Geometry check sheet. Reference: the model listing, model coordinates, mm. Face numbers are marked on the shaded views. A direction names the side the tool comes from. Coordinates: 2 decimals unless noted, no trailing zeros. Order: outer loops, then holes, each group sorted by start corner. A loop starts at its lowest first (then second) coordinate and runs counter-clockwise, first axis right, second up. Notation, with made-up numbers: (0.25, 82.25) -> (19.25, 82.25) arc R24 cw to (19.25, 108.25) -> close; hole circle Ø9 at (-32.5, 72). An arc over 180 degrees is marked (long way). Answer as CSV lines item,"result". Start each with the question number.
Autodesk Inventor part; units mm, degrees
ref_plane "YZ Plane" through (0, 0, 0) normal (1, 0, 0) x (0, 1, 0)
ref_plane "XZ Plane" through (0, 0, 0) normal (0, 1, 0) x (-1, 0, 0)
ref_plane "XY Plane" through (0, 0, 0) normal (0, 0, 1) x (1, 0, 0)
sketch "Sketch1" plane through (0, 0, 0) normal (0, 0, 1) x (1, 0, 0)
  line L0 (0, 0) -> (44, 0)
  line L1 (44, 0) -> (44, -20)
  line L2 (44, -20) -> (0, -20)
  line L3 (0, -20) -> (0, 0)
  dimension "d0" = 44
  dimension "d1" = 20
extrude "Extrusion1" add sketch "Sketch1" along normal mid plane 2
sketch "Sketch2" plane through (42, 0, -1) normal (1, 0, 0) x (0, 1, 0)
  line L0 (-20, 0) -> (0, 0)
  line L1 (0, 0) -> (0, 28)
  line L2 (0, 28) -> (-20, 28)
  line L3 (-20, 28) -> (-20, 0)
edge flange "Flange1" height 28 angle 90 thickness 2 bend radius 2 thickness toward (1, 0, 0) relief tear relief width 2 relief depth 1 corner gap 2 corner form 0 edges at (44, -10, 1) (0, -10, 1) wall of the first edge with corners at (42, -20, -1) (42, 0, -1) (42, 0, 27) (42, -20, 27)
bend "Bend1"
corner "Corner1"
sketch "Sketch3" plane through (44, -20, 27) normal (1, 0, 0) x (0, 0, -1)
  line L0 (24, 0) -> (0, 0)
  line L1 (0, 0) -> (0, 20)
  line L2 (0, 0) -> (0, 20)
  line L3 (0, 20) -> (10, 20)
  line L4 (0, 20) -> (24, 20)
  line L5 (0, 0) -> (10, 0)
  arc A0 (10, 20) -> (10, 0) centre (10, 10) ccw
  circle A1 centre (10, 10) radius 4
  point P0 (27, 20)
  point P1 (0, 10)
  dimension "d15" = 10
  dimension "d16" = 8
extrude "Cut1" cut sketch "Sketch3" against normal blind 2
sketch "Sketch4" plane through (0, -20, 27) normal (-1, 0, 0) x (0, 0, 1)
  circle A0 centre (-10, 10) radius 4
  circle A1 centre (-10, 10) radius 4
  point P0 (-27, 20)
extrude "Cut2" cut sketch "Sketch4" against normal blind 2
sketch "Sketch5" plane through (0, 0, -1) normal (0, 0, -1) x (-1, 0, 0)
  line L0 (-4, -20) -> (-4, 0)
  line L1 (-4, 0) -> (-40, 0)
  line L2 (-40, -20) -> (-4, -20)
  line L3 (-40, 0) -> (-40, -20)
  circle A0 centre (-22, -10) radius 4.5
  point P0 (0, 0)
  dimension "d21" = 9
  dimension "d22" = 18
  dimension "d23" = 10
extrude "Extrusion2" add sketch "Sketch5" along normal blind 0.1 contours A0
equation "\"d17\" = Thickness"
equation "\"d19\" = Thickness"
equation "\"d4\" = Thickness"
equation "\"d5\" = BendReliefWidth"
equation "\"d6\" = BendReliefDepth"
equation "\"d7\" = MinimumRemnant"
equation "\"d8\" = TransitionRadius"
equation "\"d11\" = BendRadius"
equation "\"d12\" = CornerReliefSize"
equation "\"d13\" = GapSize"
equation "\"d14\" = JacobiRadiusSize"
equation "\"BendRadius\" = Thickness"
equation "\"BendReliefWidth\" = Thickness"
equation "\"BendReliefDepth\" = 0.5 * Thickness"
equation "\"CornerReliefSize\" = 4 * Thickness"
equation "\"MinimumRemnant\" = 2 * Thickness"
equation "\"TransitionRadius\" = BendRadius"
equation "\"JacobiRadiusSize\" = BendRadius"
equation "\"GapSize\" = Thickness"
properties part number "SHEET_METAL2"
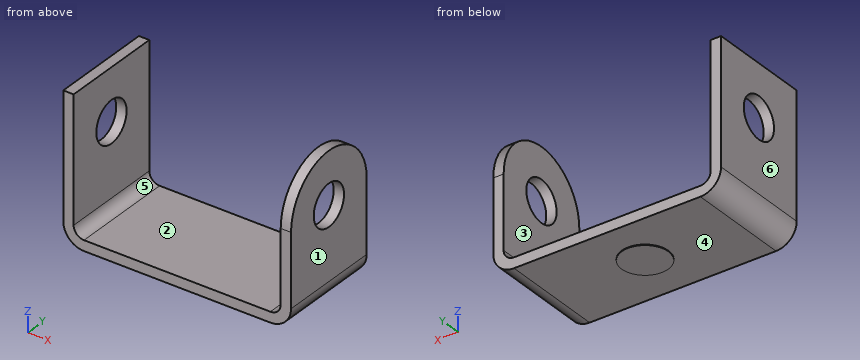
Q1. Sectioned sample at C-C, the plane y = -2. Record the cut outline in (x, z), then the cut area to 3 significant figures.
Q2. Sectioned sample at D-D, the plane z = 16.5. Record the cut outline in (x, y), then the cut area to 3 significant figures.
Q3. Thickness scan on L1, parallel to X at y = -15, z = 5.5; L2, parallel to Y at x = 1.65, z = 17; L3, parallel to Z at x = 19.5, y = -13. Record the ranges inside material, lowest first.
Q4. Sectioned sample at B-B, the plane y = -10. Record the cut outline in (x, z), then the cut area to 3 significant figures.
Q5. Go/stop test with flat-tipped pins: pin 1 Ø9 at (y, z) = (-10, 17) entering from +X; pin 2 Ø1 at (x, y) = (30.5, -13) entering from +Z. Record where each tip stops, or that it passes through.
Q6. Sectioned sample at A-A, the plane z = 8.5. Record the cut outline in (x, y), then the cut area to 3 significant figures.
Q7. Access from +Z, -Z, +X, -X, +Y, -Y to the whole of each face (thin tool, end or side, straight path). Record for the marked faces 5 and 6.
Q8. Release check for a two-part mould opening along X. For the marked faces 1, 2, 3 and 4 record: released by +X, released by -X, zero draft, split by the parting line, or undercut.
Geometry results:
1,outline,"(0, 3) arc R4 ccw to (4, -1) -> (40, -1) arc R4 ccw to (44, 3) -> (44, 23) -> (42, 23) -> (42, 3) arc R2 cw to (40, 1) -> (4, 1) arc R2 cw to (2, 3) -> (2, 27) -> (0, 27) -> close"
1,area,"179 mm^2"
2,outline,"(0, -20) -> (2, -20) -> (2, -13.97) -> (0, -13.97) -> close; (0, -6.03) -> (2, -6.03) -> (2, 0) -> (0, 0) -> close; (42, -20) -> (44, -20) -> (44, -13.97) -> (42, -13.97) -> close; (42, -6.03) -> (44, -6.03) -> (44, 0) -> (42, 0) -> close"
2,area,"48.3 mm^2"
3,L1,"x = 0 to 2, 42 to 44"
3,L2,"y = -20 to -14, -6 to 0"
3,L3,"z = -1.1 to 1"
4,outline,"(0, 3) arc R4 ccw to (4, -1) -> (17.5, -1) -> (17.5, -1.1) -> (26.5, -1.1) -> (26.5, -1) -> (40, -1) arc R4 ccw to (44, 3) -> (44, 13) -> (42, 13) -> (42, 3) arc R2 cw to (40, 1) -> (4, 1) arc R2 cw to (2, 3) -> (2, 13) -> (0, 13) -> close; (0, 21) -> (2, 21) -> (2, 27) -> (0, 27) -> close; (42, 21) -> (44, 21) -> (44, 27) -> (42, 27) -> close"
4,area,"156 mm^2"
5,pin 1,"stops at x = 44"
5,pin 2,"stops at z = 1"
6,outline,"(0, -20) -> (2, -20) -> (2, 0) -> (0, 0) -> close; (42, -20) -> (44, -20) -> (44, 0) -> (42, 0) -> close"
6,area,"80.0 mm^2"
7,face 5,"+Z, +Y, -Y"
7,face 6,"+Z, -Z, -X, +Y, -Y"
8,face 1,"released by +X"
8,face 2,"undercut"
8,face 3,"undercut"
8,face 4,"zero draft"
